Design review of the part built by this model. Coordinates are the model's own, in mm. Coordinates: 2 decimals unless noted, no trailing zeros. Write each loop counter-clockwise with the first axis right and the second up, starting at its lowest first coordinate (ties: lowest second). Pieces come first, ordered by that corner, then holes. Notation, with made-up numbers: (-4, 3.5) -> (7, 3.5) arc R16 ccw to (7, 25.5) -> close; hole circle Ø8 at (-25.75, 63). An arc over 180 degrees is marked (long way). Return JSON: item names as keys, results as strings. Group by question number.
from build123d import *

# Parameters (mm, degrees)
BOSS_EXTRUDE1_DEPTH = 2
SKETCH3_R           = 1.5
CUT_EXTRUDE1_DEPTH  = 2
CIRPATTERN1_COUNT   = 6


with BuildPart() as part:
    # Sketch2 → Boss-Extrude1 (new body)
    with BuildSketch(Plane.XY):
        Polygon((35, -60.621778265), (70, 0), (35, 60.621778265), (-35, 60.621778265), (-70, 0), (-35, -60.621778265), align=None)
    extrude(amount=BOSS_EXTRUDE1_DEPTH)

    # Sketch3 → Cut-Extrude1 (cut)
    with BuildSketch(Plane.XY):
        with Locations((27.5, -47.631397208)):
            Circle(SKETCH3_R)
        with Locations((20, -34.641016151)):
            Circle(SKETCH3_R)
    cut_extrude1 = extrude(amount=CUT_EXTRUDE1_DEPTH, mode=Mode.SUBTRACT)

    # CirPattern1: Cut-Extrude1 ×6 about axis
    cirpattern1_axis = Axis((-0.026403444, 0.045732107, 0), (0, 0, 1))
    for i in range(1, CIRPATTERN1_COUNT):
        add(cut_extrude1.rotate(cirpattern1_axis, i * 360 / CIRPATTERN1_COUNT), mode=Mode.SUBTRACT)


solid = part.part
Q1. We need section B-B on y = 38. Write out the cut boundary in (x, z), plus the area to 3 significant figures.
Q2. We need section C-C on x = -60. Write out the cut boundary in (y, z).
Q3. We need section A-A on z = 0.3. State how many separate pieces and enclosed holes the cut face has, plus the area to 3 significant figures.
Q4. Wall thickness on L1, parallel to Y at x = 20, z = 0.6; L2, parallel to Y at x = 27.5, z = 1.65; L3, parallel to X at y = -47, z = 0.2: over which ranges is each line inside the solid? List them lowest first.
Q5. The part is to be moulded in two halves that separate along X. For faces 1 (the cylindrical face through (-28.984, 47.272, 0.986)), 2 (the cylindrical face through (28.19, 46.39, 0.99)), 3 (the flat face through (52.745, 29.887, 0.986)), 4 (the flat face through (-52.255, 30.735, 0.986)), say which applies: +X half, -X half, draft (parallel to the pull), parting line (faces both ways), or undercut.
Findings below:
{
 "1": {"outline": "(-48.06, 0) -> (48.06, 0) -> (48.06, 2) -> (-48.06, 2) -> close", "area": "192 mm^2"},
 "2": {"outline": "(-17.32, 0) -> (17.32, 0) -> (17.32, 2) -> (-17.32, 2) -> close"},
 "3": {"separate pieces": "1", "enclosed holes": "12", "area": "12,600 mm^2"},
 "4": {"L1": "y = -60.62 to -36.14, -33.14 to 33.23, 36.23 to 60.62", "L2": "y = -60.62 to -49.13, -46.13 to 46.22, 49.22 to 60.62", "L3": "x = -42.86 to -28.91, -26.19 to 26.14, 28.86 to 42.86"},
 "5": {"face 1": "undercut", "face 2": "undercut", "face 3": "+X half", "face 4": "-X half"}
}
